The model under review builds one solid part; all positions refer to its coordinate system, in mm. A direction names the side the tool comes from. Coordinates: 2 decimals unless noted, no trailing zeros. Loops run counter-clockwise (first coordinate to the right, second up) from the corner with the lowest first, then second, coordinate; pieces in that order, holes last. Notation, with made-up numbers: M 45,28 L 70,28 A26 cw 70,46 Z; hole C -30,15.25 d3. An arc over 180 degrees is marked long. Write item = value, one per line. Start each with the question number.
Q1. We need section B-B on y = 87. Give the boundary of the cut face in (x, z).
Q2. Clearance check with flat-ended pins moving along their axes: pin 1 Ø3 at (x, z) = (-152.4, 3.175) entering from -Y; pin 2 Ø10 at (y, z) = (84, 97.5) entering from -X; pin 3 Ø6 at (y, z) = (18, 64) entering from -X; pin 4 Ø6 at (y, z) = (30, 127.5) entering from -X. State where each tip first meets the part, or that it passes through.
Q3. For faces 1 (the face through (154, -1.228, 106)), 2 (the face through (-158, 107.516, 106)), 3 (the face through (-158, 106.722, 106)), list the 3-axis set-ups (+Z, -Z, +X, -X, +Y, -Y) from which the entire face can be reached by the end or side of a thin tool; tool diameter is ignored.
Q4. Wall thickness on probe 1 along Z at (x, y) = (-152.4, 106.95); probe 2 along Y at (x, z) = (-60.5, 148); probe 3 along Y at (x, z) = (-113, 109.5): over which ranges is each line inside the solid? List them lowest first.
Q5. We need section C-C on x = 140. Give the boundary of the cut face in (y, z), and give its area (3 significant figures).
Autodesk Inventor part; units mm, degrees
ref_plane "Work Plane1" through (0, 0, 0) normal (0, 0, 1) x (1, 0, 0)
ref_plane "YZ Plane" through (0, 0, 0) normal (1, 0, 0) x (0, 1, 0)
ref_plane "XZ Plane" through (0, 0, 0) normal (0, 1, 0) x (-1, 0, 0)
ref_plane "Work Plane1" through (0, 0, 0) normal (0, 0, 1) x (1, 0, 0)
sketch "Sketch1" plane through (0, 0, 0) normal (0, 0, 1) x (1, 0, 0)
  line L0 (165.1, 107.5162) -> (-165.1, 107.5162) construction
  line L1 (-165.1, 107.5162) -> (-165.1, 110.6912) construction
  line L2 (165.1, 110.6912) -> (-165.1, 110.6912) construction
  line L3 (165.1, 107.5162) -> (165.1, 110.6912) construction
  line L4 (161.925, -1.2275) -> (161.925, 14.6475) construction
  line L5 (161.925, 14.6475) -> (161.1313, 14.6475) construction
  line L6 (161.1313, 14.6475) -> (161.1313, -0.4338) construction
  line L7 (161.1313, -0.4338) -> (146.05, -0.4338) construction
  line L8 (146.05, -0.4338) -> (146.05, -1.2275) construction
  line L9 (146.05, -1.2275) -> (161.925, -1.2275) construction
  line L10 (-153.9875, 110.6912) -> (-150.8125, 110.6912) construction
  line L11 (161.925, -1.2275) -> (146.05, -1.2275)
  arc A0 (-23.8125, 60.9948) -> (-150.8125, 107.5162) centre (-150.8125, -89.0948) ccw
  arc A1 (-23.8125, 60.9948) -> (146.05, -1.2275) centre (146.05, 261.7398) ccw
  line L12 (-150.8125, 110.6912) -> (-150.8125, 107.5162) construction
  line L13 (-150.8125, 107.5162) -> (-165.1, 107.5162)
  arc A2 (-24.3252, 60.3889) -> (-150.8125, 106.7225) centre (-150.8125, -89.0948) ccw
  arc A3 (-24.3252, 60.3889) -> (146.05, -2.0213) centre (146.05, 261.7398) ccw
  line L14 (146.05, -2.0213) -> (161.925, -2.0213)
  line L15 (-165.1, 107.5162) -> (-165.1, 106.7225)
  line L16 (-165.1, 106.7225) -> (-150.8125, 106.7225)
  line L17 (161.925, -1.2275) -> (161.925, -2.0213)
  point P0 (0, 0)
  dimension "d8" = 127
  dimension "d9" = 0.7937
extrude "Extrusion1" add sketch "Sketch1" along normal blind 215.9
sketch "Sketch2" plane through (-165.1, 106.7225, 0) normal (0, -1, 0) x (1, 0, 0)
  circle A0 centre (12.7, 3.175) radius 1.5875
  circle A1 centre (12.7, 104.775) radius 1.5875
  circle A2 centre (12.7, 206.375) radius 1.5875
  line L0 (14.2875, 0) -> (0, 0)
  line L1 (14.2875, 0) -> (14.2875, 215.9)
  line L2 (0, 215.9) -> (14.2875, 215.9)
  line L3 (0, 0) -> (0, 215.9)
  point P0 (165.1, 0)
extrude "Extrusion2" cut sketch "Sketch2" against normal through all contours A0 | A1 | A2
sketch "Sketch3" plane through (146.05, -1.2275, 0) normal (0, 1, 0) x (1, 0, 0)
  circle A0 centre (7.5406, -198.5968) radius 1.5875
  circle A1 centre (7.5406, -27.1468) radius 1.5875
  point P0 (-146.05, 0)
extrude "Extrusion3" cut sketch "Sketch3" against normal through all
properties part number "Bounce Polycarbonate Flap" material "Polycarbonate, Clear"
Returned:
q1.outline = M -65.17,0 L -63.37,0 L -63.37,215.9 L -65.17,215.9 Z
q2.pin_1 = through
q2.pin_2 = -69.41
q2.pin_3 = 38.28
q2.pin_4 = 14.72
q3.face_1 = +Z, -Z, +X, +Y
q3.face_2 = +Z, -Z, +X, -X, +Y
q3.face_3 = +Z, -Z, -X, -Y
q4.probe_1 = 0 to 1.59, 4.76 to 103.19, 106.36 to 204.79, 207.96 to 215.9
q4.probe_2 = 84.65 to 85.55
q4.probe_3 = 103.04 to 103.85
q5.outline = M -1.95,0 L -1.16,0 L -1.16,215.9 L -1.95,215.9 Z
q5.area = 171 mm^2
